```python
from build123d import *

# Parameters (mm, degrees)
F0_R     = 38.1
F1_DEPTH = 6.35
F2_R     = 31.75
F2_R_2   = 25.654
F3_DEPTH = 152.4
F4_R     = 3.175
F5_DEPTH = 25.4
F6_SIZE  = 5.08


with BuildPart() as f1:
    # F0 (on Top) → F1 (new body)
    with BuildSketch(Plane.XY):
        Circle(F0_R)
    extrude(amount=F1_DEPTH)

    # F2 (on face) → F3 (join)
    with BuildSketch(Plane.XY.offset(6.35)):
        Circle(F2_R)
        Circle(F2_R_2, mode=Mode.SUBTRACT)
    extrude(amount=F3_DEPTH)

    # F4 (on face) → F5 (cut)
    with BuildSketch(Plane.XY.offset(6.35)):
        Circle(F4_R)
    extrude(amount=-F5_DEPTH, mode=Mode.SUBTRACT)

    # F6
    f6_edges = [f1.edges().sort_by_distance(p)[0] for p in [
        (-25.654, 0, 158.75),
    ]]
    chamfer(f6_edges, length=F6_SIZE)


solid = f1.part
```
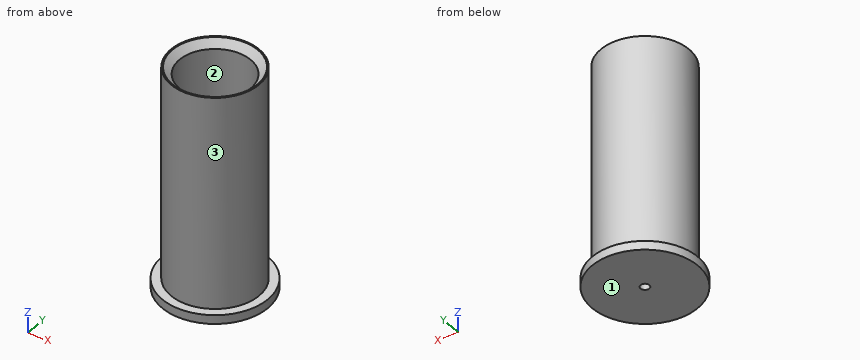
The listing builds one solid part. Answer for the finished solid, in the listing's coordinates (mm). Face numbers are marked on the shaded views. Round coordinates to 2 decimals unless told otherwise and drop trailing zeros. Loops run counter-clockwise (first coordinate to the right, second up) from the corner with the lowest first, then second, coordinate; pieces in that order, holes last. Notation, with made-up numbers: (31, 75) -> (43, 75) arc R18 cw to (43, 80) -> close; hole circle Ø9 at (-26.5, 29.25). An arc over 180 degrees is marked (long way). Use one line per item in the form item = value.
1. The part is cut by section C-C on z = 55.5. Determine the outline of the cut face in (x, y).
Answer key:
outline = circle Ø63.5 at (0, 0); hole circle Ø51.31 at (0, 0)
2. Flat-ended cylindrical pins translate along their axes: pin 1 Ø12 at (x, y) = (-6, 18) entering from +Z; pin 2 Ø4 at (x, z) = (29, 25.5) entering from -Y; pin 3 Ø3 at (x, z) = (-10.5, 33) entering from -Y. Find the tip coordinate at first contact, or state that the pin passes through.
Answer key:
pin_1 = 6.35
pin_2 = -16.71
pin_3 = -30.45
3. The part is cut by section A-A on y = 0. Determine the outline of the cut face in (x, z) (3 decimals), and give its area (3 significant figures).
Answer key:
outline = (-38.1, 0) -> (-3.175, 0) -> (-3.175, 6.35) -> (-25.654, 6.35) -> (-25.654, 153.67) -> (-30.734, 158.75) -> (-31.75, 158.75) -> (-31.75, 6.35) -> (-38.1, 6.35) -> close; (3.175, 0) -> (38.1, 0) -> (38.1, 6.35) -> (31.75, 6.35) -> (31.75, 158.75) -> (30.734, 158.75) -> (25.654, 153.67) -> (25.654, 6.35) -> (3.175, 6.35) -> close
area = 2,280 mm²
4. Find the intervals of material crossed by probe 1 along X at (y, z) = (-0.5, 99), in increasing order. Write a range as [from, to].
Answer key:
probe_1 = [-31.75, -25.65], [25.65, 31.75]
5. For a pull along Y with two mould halves and no side action, classify the marked faces 1, 2 and 3 as released by +Y, released by -Y, zero draft, split by the parting line, or undercut.
Answer key:
face_1 = zero draft
face_2 = undercut
face_3 = split by the parting line
